CAD build for the part. Positions are in the model's coordinates, mm. A direction names the side the tool comes from. Coordinates: 2 decimals unless noted, no trailing zeros. Order: outer loops, then holes, each group sorted by start corner. A loop starts at its lowest first (then second) coordinate and runs counter-clockwise, first axis right, second up. Notation, with made-up numbers: (17, 35) - (70, 35) arc R18 ccw to (70, 47) - close; hole circle Ø3 at (54, -24). An arc over 180 degrees is marked (long way). Write each question's results on one line, items separated by ' | '. Start each with the question number.
Q1. Which spindle directions (+Z, -Z, +X, -X, +Y, -Y) get a long thin tool onto all of the face, cutting with end or side? Do faces 1 (the cylindrical face through (-0.27, -1.22, 14.79)), 2 (the cylindrical face through (-0.3, -1.34, 30.25)). Say none if no direction does.
Q2. Wall check: probe 1 along X at (y, z) = (0.1, 18); probe 2 along X at (y, z) = (1, 5). Give the ranges that are in metal, low to high.
Q3. Band-saw the part on A-A, the plane y = 0. Write the cut outline in (x, z) (3 decimals), then the cut area to 3 significant figures.
Q4. Pin check, flat tips, straight feed: P1, Ø1.5, axis at x = 0.5, z = 12.5, coming from the +Y side; P2, Ø1.5, axis at y = 0.5, z = 11.5, coming from the +X side. Stop position of each tip, or through.
Q5. Band-saw the part on C-C, the plane z = 4.5. Write the cut outline in (x, y), then the cut area to 3 significant figures.
```python
from build123d import *

# Parameters (mm, degrees)
SKETCH2_R           = 1.25
BOSS_EXTRUDE1_DEPTH = 30
SKETCH3_R           = 1.375
BOSS_EXTRUDE2_DEPTH = 0.5
FILLET1_R           = 0.1


with BuildPart() as part:
    # Sketch2 → Boss-Extrude1 (new body)
    with BuildSketch(Plane.XY):
        Circle(SKETCH2_R)
    extrude(amount=BOSS_EXTRUDE1_DEPTH)

    # Sketch3 → Boss-Extrude2 (add)
    with BuildSketch(Plane.XY.offset(30)):
        Circle(SKETCH3_R)
    extrude(amount=BOSS_EXTRUDE2_DEPTH)

    # Fillet1
    fillet1_edges = [part.edges().sort_by_distance(p)[0] for p in [
        (-1.375, 0, 30),
        (-1.375, 0, 30.5),
    ]]
    fillet(fillet1_edges, radius=FILLET1_R)


solid = part.part
```
Results below:
1) face 1: -Z | face 2: +Z, -Z
2) probe 1: x = -1.25 to 1.25 | probe 2: x = -0.75 to 0.75
3) outline: (-1.375, 30.1) arc R0.1 ccw to (-1.275, 30) - (-1.25, 30) - (-1.25, 0) - (1.25, 0) - (1.25, 30) - (1.275, 30) arc R0.1 ccw to (1.375, 30.1) - (1.375, 30.4) arc R0.1 ccw to (1.275, 30.5) - (-1.275, 30.5) arc R0.1 ccw to (-1.375, 30.4) - close | area: 76.4 mm²
4) P1: stops at y = 1.25 | P2: stops at x = 1.25
5) outline: circle Ø2.5 at (0, 0) | area: 4.91 mm²
